For this review, take the finished solid that the model builds, in its own axes (mm). A direction names the side the tool comes from. Give positions to 0.01 mm unless a question says otherwise; leave off trailing zeros. Order: outer loops, then holes, each group sorted by start corner. A loop starts at its lowest first (then second) coordinate and runs counter-clockwise, first axis right, second up.
from build123d import *

# Parameters (mm, degrees)
SKETCH1_W           = 200
SKETCH1_H           = 120
SKETCH1_R           = 5
BOSS_EXTRUDE3_DEPTH = 1.5
SKETCH2_W           = 120
SKETCH2_H           = 13
BOSS_EXTRUDE4_DEPTH = 1
SKETCH3_W           = 202
SKETCH3_H           = 13
BOSS_EXTRUDE6_DEPTH = 1


with BuildPart() as part:
    # Sketch1 → Boss-Extrude3 (new, symmetric)
    with BuildSketch(Plane(origin=(0, 0, 0), x_dir=(1, 0, 0), z_dir=(0, 1, 0))):
        Rectangle(SKETCH1_W, SKETCH1_H)
        with Locations(Location((-80, 40, 0), (0, 0, 270))):
            Circle(SKETCH1_R, mode=Mode.SUBTRACT)
        with Locations(Location((80, 40, 0), (0, 0, 90))):
            Circle(SKETCH1_R, mode=Mode.SUBTRACT)
        with Locations(Location((80, -40, 0), (0, 0, 270))):
            Circle(SKETCH1_R, mode=Mode.SUBTRACT)
        with Locations(Location((-80, -40, 0), (0, 0, 90))):
            Circle(SKETCH1_R, mode=Mode.SUBTRACT)
    extrude(amount=BOSS_EXTRUDE3_DEPTH, both=True)

    # Sketch2 → Boss-Extrude4 (add)
    with BuildSketch(Plane.ZY.offset(100)):
        with Locations((0, 5)):
            Rectangle(SKETCH2_W, SKETCH2_H)
    boss_extrude4 = extrude(amount=BOSS_EXTRUDE4_DEPTH)

    # Mirror1: Boss-Extrude4 across plane
    add(boss_extrude4.mirror(Plane(origin=(0, 0, 0), x_dir=(0, 0, 1), z_dir=(1, 0, 0))))

    # Sketch3 → Boss-Extrude6 (add)
    with BuildSketch(Plane(origin=(0, 0, -60), x_dir=(-1, 0, 0), z_dir=(0, 0, -1))):
        with Locations((0, 5)):
            Rectangle(SKETCH3_W, SKETCH3_H)
    boss_extrude6 = extrude(amount=BOSS_EXTRUDE6_DEPTH)

    # Mirror2: Boss-Extrude6 across plane
    add(boss_extrude6.mirror(Plane.XY))


solid = part.part
1) We need section C-C on y = 6.5. Give the boundary of the cut face in (x, z), then the cut area to 3 significant figures.
Answer sheet:
outline: (-101, -61) - (101, -61) - (101, 61) - (-101, 61) - close; hole (-100, -60) - (100, -60) - (100, 60) - (-100, 60) - close
area: 644 mm2
2) We need section B-B on x = 80. Give the boundary of the cut face in (y, z).
Answer sheet:
outline: (-1.5, -61) - (11.5, -61) - (11.5, -60) - (1.5, -60) - (1.5, -45) - (-1.5, -45) - close; (-1.5, -35) - (1.5, -35) - (1.5, 35) - (-1.5, 35) - close; (-1.5, 45) - (1.5, 45) - (1.5, 60) - (11.5, 60) - (11.5, 61) - (-1.5, 61) - close
3) Tool access review of faces 4 (the face through (100, 7, -1)), 5 (the face through (1, 5, 61)): name each direction out of +Z, -Z, +X, -X, +Y, -Y from which nothing blocks a thin tool from reaching the whole face with its end or side.
Answer sheet:
face 4: +Y
face 5: +Z, +X, -X, +Y, -Y
4) We need section A-A on z = -37. Give the boundary of the cut face in (x, y), then the cut area to 3 significant figures.
Answer sheet:
outline: (-101, -1.5) - (-84, -1.5) - (-84, 1.5) - (-100, 1.5) - (-100, 11.5) - (-101, 11.5) - close; (-76, -1.5) - (76, -1.5) - (76, 1.5) - (-76, 1.5) - close; (84, -1.5) - (101, -1.5) - (101, 11.5) - (100, 11.5) - (100, 1.5) - (84, 1.5) - close
area: 578 mm2
5) To check wall thickness, follow line 1 (X direction, y = -0.1, z = -40); line 2 (X direction, y = 2, z = 50.5); line 3 (Z direction, x = -27, y = 4.25). State the ranges of each line that lie inside material, in increasing order.
Answer sheet:
line 1: x = -101 to -85, -75 to 75, 85 to 101
line 2: x = -101 to -100, 100 to 101
line 3: z = -61 to -60, 60 to 61
6) Clearance check with a flat-ended pin moving along its axis: pin 1 (4 mm diameter, centred on x = 40.5, z = -42.5, fed in from +Y). State where the tip first meets the part, or that it passes through.
Answer sheet:
pin 1: stops at y = 1.5
7) Draft analysis for pull direction Z (two halves, no side actions). For faces 1 (the face through (1, 5, -61)), 2 (the face through (-1, 1.5, -1)), 3 (the face through (-101, 5, -1)), state which applies: +Z half, -Z half, draft (parallel to the pull), parting line (faces both ways), or undercut.
Answer sheet:
face 1: -Z half
face 2: undercut
face 3: draft
8) We need section D-D on z = 11. Give the boundary of the cut face in (x, y).
Answer sheet:
outline: (-101, -1.5) - (101, -1.5) - (101, 11.5) - (100, 11.5) - (100, 1.5) - (-100, 1.5) - (-100, 11.5) - (-101, 11.5) - close
